Source: CAD feature listing. Evaluate the final solid. Frame: model axes, mm. A direction names the side the tool comes from. Coordinates: 2 decimals unless noted, no trailing zeros. Loops run counter-clockwise (first coordinate to the right, second up) from the corner with the lowest first, then second, coordinate; pieces in that order, holes last. Notation, with made-up numbers: (78.5, -10) -> (109.5, -10) arc R26 ccw to (109.5, 4) -> close; hole circle Ø11 at (1, 16). An arc over 180 degrees is marked (long way). Answer as CSV lines item,"result".
from build123d import *

# Parameters (mm, degrees)
BOSS_EXTRUDE1_DEPTH = 6.35
FILLET1_R           = 9.525
SKETCH2_R           = 1.5
CUT_EXTRUDE1_DEPTH  = 154.324560084


with BuildPart() as part:
    # Sketch1 → Boss-Extrude1 (new body)
    with BuildSketch(Plane(origin=(0, 0, 0), x_dir=(1, 0, 0), z_dir=(0, 1, 0))):
        Polygon((-120.65, -62.865), (-120.65, 43.815), (120.65, 43.815), (120.65, -62.865), (139.7, -62.865), (139.7, 62.865), (-139.7, 62.865), (-139.7, -62.865), align=None)
    extrude(amount=-BOSS_EXTRUDE1_DEPTH)

    # Fillet1
    fillet1_edges = [part.edges().sort_by_distance(p)[0] for p in [
        (120.65, -3.175, -43.815),
        (-120.65, -3.175, -43.815),
    ]]
    fillet(fillet1_edges, radius=FILLET1_R)

    # Sketch2 → Cut-Extrude1 (cut, through all)
    with BuildSketch(Plane(origin=(0, 0, 0), x_dir=(1, 0, 0), z_dir=(0, 1, 0))):
        with Locations(Location((-133.35, -50.165, 0), (0, 0, 270))):
            Circle(SKETCH2_R)
        with Locations(Location((-127, -56.515, 0), (0, 0, 270))):
            Circle(SKETCH2_R)
        with Locations(Location((-132.42006403, 55.58506403, 0), (0, 0, 270))):
            Circle(SKETCH2_R)
        with Locations(Location((-125.140128061, 48.305128061, 0), (0, 0, 270))):
            Circle(SKETCH2_R)
        with Locations(Location((125.140128061, 48.305128061, 0), (0, 0, 90))):
            Circle(SKETCH2_R)
        with Locations(Location((132.42006403, 55.58506403, 0), (0, 0, 90))):
            Circle(SKETCH2_R)
        with Locations(Location((127, -56.515, 0), (0, 0, 90))):
            Circle(SKETCH2_R)
        with Locations(Location((133.35, -50.165, 0), (0, 0, 90))):
            Circle(SKETCH2_R)
    extrude(amount=-CUT_EXTRUDE1_DEPTH, mode=Mode.SUBTRACT)


solid = part.part
(1) Cut plane D-D (x = 115). Return the cut outline in (y, z) (3 decimals).
Computed values:
outline,"(-6.35, -62.865) -> (0, -62.865) -> (0, -42.991) -> (-6.35, -42.991) -> close"
(2) Cut plane B-B (y = -1.75). State how many separate pieces and enclosed holes the cut face has, then the cut area to 3 significant figures.
Computed values:
separate pieces,"1"
enclosed holes,"8"
area,"9,370 mm^2"
(3) Cut plane A-A (z = -0.5). Return the cut outline in (x, y), then the cut area to 3 significant figures.
Computed values:
outline,"(-139.7, -6.35) -> (-120.65, -6.35) -> (-120.65, 0) -> (-139.7, 0) -> close; (120.65, -6.35) -> (139.7, -6.35) -> (139.7, 0) -> (120.65, 0) -> close"
area,"242 mm^2"
(4) Material intervals for L1, parallel to Z at x = 127, y = -2.75 (3 decimals); L2, parallel to X at y = -4.5, z = 21.5; L3, parallel to Z at x = 7, y = -5.5 (3 decimals), sorted ascending. Write a range as [from, to].
Computed values:
L1,"[-62.865, 55.015], [58.015, 62.865]"
L2,"[-139.7, -120.65], [120.65, 139.7]"
L3,"[-62.865, -43.815]"
(5) Access query for faces 1 (the flat face through (130, -3, 62.865)), 2 (the cylindrical face through (-117.934, -3.219, -40.951)). Directions: +Z, -Z, +X, -X, +Y, -Y. A direction counts if a zero-diameter tool reaches every point of the face in a straight line with its end or side. Return the directions, or none.
Computed values:
face 1,"+Z, +X, -X, +Y, -Y"
face 2,"+Z, +Y, -Y"
(6) Cut plane C-C (x = -65.5). Return the cut outline in (y, z) (3 decimals).
Computed values:
outline,"(-6.35, -62.865) -> (0, -62.865) -> (0, -43.815) -> (-6.35, -43.815) -> close"
(7) Pin query (flat end, axial travel): pin 1 Ø2.5 at (x, z) = (133.35, 50.165) entering from -Y; pin 2 Ø5 at (x, z) = (127, 56.515) entering from -Y; pin 3 Ø1.9 at (x, y) = (2, -1.5) entering from +Z (3 decimals). Return the tip coordinate at first contact, or that it passes through.
Computed values:
pin 1,"through"
pin 2,"y = -6.35"
pin 3,"z = -43.815"
(8) Draft query along X for faces 3 (the flat face through (-139.7, -3, -1)), 4 (the flat face through (-1, -6.35, -47)), 5 (the flat face through (-2, -3, -43.815)). Return one class per face: released by +X, released by -X, zero draft, split by the parting line, or undercut.
Computed values:
face 3,"released by -X"
face 4,"zero draft"
face 5,"undercut"
